Autodesk Inventor part; units mm, degrees
ref_plane "Work Plane2" through (3.35, 0, 0) normal (0, 0, -1) x (1, 0, 0)
ref_plane "YZ Plane" through (0, 0, 0) normal (1, 0, 0) x (0, 1, 0)
ref_plane "XZ Plane" through (0, 0, 0) normal (0, 1, 0) x (-1, 0, 0)
sketch "Sketch1" plane through (0, 0, 0) normal (0, 0, 1) x (1, 0, 0)
  line L0 (1.88, 0) -> (10, 0)
  line L1 (10, 0) -> (10, 2)
  line L2 (10, 2) -> (3.6, 2)
  line L3 (3.6, 2) -> (3.1706, 1.7853)
  line L4 (3.1706, 1.7853) -> (2.2, 1.7853)
  line L5 (0, 3.5) -> (0, 2.11)
  line L6 (0, 2.11) -> (1.0316, 1.5957)
  line L7 (1.0316, 1.5957) -> (1.88, 0)
  line L8 (-2, 0) -> (12, 0)
  line L9 (0, -0.7) -> (0, 4.2)
  line L10 (0, 3.5) -> (0.4853, 3.5)
  line L11 (0.4853, 3.5) -> (2.2, 1.7853)
  line L12 (3.6, 2) -> (1.9853, 2) construction
  dimension "d1" = 6.4
  dimension "d2" = 4
  dimension "d3" = 3.5706
  dimension "d4" = 4.22
  dimension "d5" = 26.5
  dimension "d6" = 62
  dimension "d7" = 1.88
  dimension "d8" = 0.4294
  dimension "d12" = 7
  dimension "d13" = 45
  dimension "d15" = 10
  dimension "d24" = 2.2
revolve "Body" add sketch "Sketch1" angle 360 about axis through (1.88, 0, 0) along (1, 0, 0) contours L7 L6 L5 L10 L11 L4 L3 L2 L1 L0
sketch "Sketch2" plane through (0, 0, 0) normal (-1, 0, 0) x (0, 0, 1)
  line L0 (0, 2.11) -> (0, 0) construction
  line L1 (0, 0) -> (2.11, 0) construction
  arc A0 (0.633, 0) -> (0, 0.633) centre (0, 0) ccw construction
  arc A1 (0.7385, 0) -> (0, 0.7385) centre (0, 0) ccw construction
  arc A2 (2.0511, 0.495) -> (0.495, 2.0511) centre (0, 0) ccw
  line L2 (0, 0) -> (1.492, 1.492) construction
  line L3 (0.495, 2.0511) -> (0.3793, 0.6337)
  line L4 (2.0511, 0.495) -> (0.6337, 0.3793)
  arc A3 (0.495, 2.0511) -> (0, 2.11) centre (0, 0) ccw
  arc A4 (2.11, 0) -> (2.0511, 0.495) centre (0, 0) ccw
  line L5 (0, -4.9) -> (0, 4.9)
  line L6 (-4.9, 0) -> (4.9, 0)
  arc A5 (0.495, -2.0511) -> (2.0511, -0.495) centre (0, 0) ccw
  line L7 (0.495, -2.0511) -> (0.3793, -0.6337)
  line L8 (2.0511, -0.495) -> (0.6337, -0.3793)
  arc A6 (0, -2.11) -> (0.495, -2.0511) centre (0, 0) ccw
  arc A7 (2.0511, -0.495) -> (2.11, 0) centre (0, 0) ccw
  arc A8 (-0.495, 2.0511) -> (-2.0511, 0.495) centre (0, 0) ccw
  line L9 (-0.495, 2.0511) -> (-0.3793, 0.6337)
  line L10 (-2.0511, 0.495) -> (-0.6337, 0.3793)
  arc A9 (0, 2.11) -> (-0.495, 2.0511) centre (0, 0) ccw
  arc A10 (-2.0511, 0.495) -> (-2.11, 0) centre (0, 0) ccw
  arc A11 (-0.495, -2.0511) -> (0, -2.11) centre (0, 0) ccw
  arc A12 (-2.0511, -0.495) -> (-0.495, -2.0511) centre (0, 0) ccw
  arc A13 (-2.11, 0) -> (-2.0511, -0.495) centre (0, 0) ccw
  line L11 (-2.0511, -0.495) -> (-0.6337, -0.3793)
  line L12 (-0.495, -2.0511) -> (-0.3793, -0.6337)
  arc A14 (0.3793, 0.6337) -> (0.6337, 0.3793) centre (0.6145, 0.6145) ccw
  arc A15 (0.6337, -0.3793) -> (0.3793, -0.6337) centre (0.6145, -0.6145) ccw
  arc A16 (-0.6337, 0.3793) -> (-0.3793, 0.6337) centre (-0.6145, 0.6145) ccw
  arc A17 (-0.3793, -0.6337) -> (-0.6337, -0.3793) centre (-0.6145, -0.6145) ccw
  point P0 (1.492, -1.492)
  point P1 (-1.492, 1.492)
  point P2 (-1.492, -1.492)
  dimension "d17" = 1.266
  dimension "d18" = 1.477
  dimension "d19" = 4.22
  dimension "d20" = 45
  dimension "d21" = 0.495
extrude "Slot" add sketch "Sketch2" against normal up to next draft 5 contours L4 A14 L3 A2 | A5 L7 A15 L8 | L9 A16 L10 A8 | A12 L11 A17 L12
fillet "Fillet1" radius 0.198 4 edges at (0, 2.11, 0) (0, 0, -2.11) (0, -2.11, 0) (0, 0, 2.11)
thread "Thread"
chamfer "Chamfer1" distance 0.4294 distance2 0.2147 1 edges at (10, -2, 0) measured on face at (10, -0.499, 0.4421)
ref_plane "Work Plane2" through (3.35, 0, 0) normal (0, 0, -1) x (1, 0, 0)
equation "\"d17\" = 0.3 * SDM"
equation "\"d18\" = 0.35 * SDM"
equation "\"d19\" = SDM"
equation "\"d21\" = 0.5 * SBR"
equation "\"d1\" = GEL"
equation "\"d2\" = GD"
equation "\"d3\" = BDM"
equation "\"d4\" = SDM"
equation "\"d7\" = INTI"
equation "\"d8\" = GAL"
equation "\"d12\" = KOD"
equation "\"d13\" = 0.5 * SEWI"
equation "\"d15\" = NLG"
equation "\"d24\" = KOH"
equation "\"d23\" = 0.2 * SBR"
equation "\"d10\" = GEL"
equation "\"d25\" = -0.5 * SPD + 0.5 * GD"
equation "\"d26\" = 0.5 * GAL"
equation "\"NLG\" = 10"
equation "\"GEL\" = 6.4"
equation "\"GAL\" = 0.61345 * PTC"
equation "\"SPD\" = NND - 1.2269 * PTC"
equation "\"KOD\" = 7"
equation "\"KOH\" = 2.2"
equation "\"SBR\" = 0.99"
equation "\"INTI\" = 1.88"
equation "\"SDM\" = 4.22"
equation "\"GD\" = NND"
equation "\"BDM\" = NND - GAL"
equation "\"SEWI\" = 90deg"
equation "\"d9\" = SDM"
equation "\"GUL\" = 0.61345 * PTC"
equation "\"TOA\" = 30deg"
equation "\"EPV\" = 4.2"
equation "\"THREADDIA\" = 4"
equation "\"RR\" = 0.4"
equation "\"PTC\" = 0.7"
equation "\"NND\" = 4"
equation "\"GD1\" = THREADDIA - 1.2269 * PTC"
properties part number "AS 1427 - M4 x 10" material "Steel, Mild"
Work out the finished part from the listing and answer in its coordinate system (mm). A direction names the side the tool comes from. Coordinates: 2 decimals unless noted, no trailing zeros. Loops run counter-clockwise (first coordinate to the right, second up) from the corner with the lowest first, then second, coordinate; pieces in that order, holes last. Notation, with made-up numbers: M -21.75,43 L 23.25,43 A20 ccw 23.25,70 Z; hole C 27.25,53.5 d3. An arc over 180 degrees is marked long. Use CSV: the item, a comma, the result in double quotes. Start each with the question number.
(1) Given pin 1 Ø1.5 at (y, z) = (-1.5, 2.5) entering from +X; pin 2 Ø2 at (x, z) = (7, 1.5) entering from -Y, each flat-ended and moving along its own axis, determine where each tip first touches the part or whether it passes through.
(2) For faces 4 (the face through (2.679, -0.387, 1.743)), 5 (the face through (0.58, -0.38, 1.25)), 6 (the face through (0.246, 3.233, -1.341)), determine the directions among +Z, -Z, +X, -X, +Y, -Y from which every point of the face is accessible in a straight line to the end or side of a thin tool.
(3) Consider line 1 (Z direction, x = 0.75, y = 1); line 2 (Z direction, x = 7, y = 1.25); line 3 (X direction, y = -2, z = -2). Determine where each line is inside the solid, lowest interval first.
(4) For a pull along Z with two mould halves and no side action, classify faces 1 (the face through (0.56, 0.01, -1.83)), 2 (the face through (7, 0, 2)), 3 (the face through (10, 0, 0)) as +Z half, -Z half, draft (parallel to the pull), parting line (faces both ways), or undercut.
(5) Find section A-A, the plane x = 7. Give the vertices of the cut face in (y, z).
Recorded:
1,pin 1,"stops at x = 1.82"
1,pin 2,"stops at y = -1.94"
2,face 4,"none"
2,face 5,"-X"
2,face 6,"+X, -X"
3,line 1,"z = -3.08 to -0.34, 0.34 to 3.08"
3,line 2,"z = -1.56 to 1.56"
3,line 3,"x = 0 to 1.16"
4,face 1,"undercut"
4,face 2,"parting line"
4,face 3,"draft"
5,outline,"C 0,0 d4"
